```python
from build123d import *

# Parameters (mm, degrees)
BOSS_EXTRUDE1_DEPTH = 15
SKETCH5_R           = 10
CUT_EXTRUDE1_DEPTH  = 15


with BuildPart() as part:
    # Sketch3 → Boss-Extrude1 (new body)
    with BuildSketch(Plane(origin=(0, 0, 0), x_dir=(0, 0, -1), z_dir=(1, 0, 0))):
        Polygon((0, 0), (120, 0), (120, 80), (80, 80), (80, 40), (40, 40), (40, 80), (0, 80), align=None)
    extrude(amount=BOSS_EXTRUDE1_DEPTH)

    # Sketch5 → Cut-Extrude1 (cut)
    with BuildSketch(Plane.ZY):
        with Locations((-100, 20)):
            Circle(SKETCH5_R)
        with Locations((-20, 20)):
            Circle(SKETCH5_R)
    extrude(amount=-CUT_EXTRUDE1_DEPTH, mode=Mode.SUBTRACT)


solid = part.part
```
Read the model definition and answer for the solid it produces. Units are mm, in the model's axes. A direction names the side the tool comes from. Give positions to 0.01 mm unless a question says otherwise; leave off trailing zeros. Write each loop counter-clockwise with the first axis right and the second up, starting at its lowest first coordinate (ties: lowest second). Pieces come first, ordered by that corner, then holes. Notation, with made-up numbers: (49, 31.5) - (96, 31.5) arc R17 ccw to (96, 36.5) - close; hole circle Ø10 at (16, 66.5). An arc over 180 degrees is marked (long way). Write item = value, one per line. Start each with the question number.
Item 1: Find section B-B (y = 20). Give the vertices of the cut face in (x, z).
Item 2: Find the intervals of material crossed by probe 1 along Z at (x, y) = (12, 17); probe 2 along Y at (x, z) = (8.25, -20); probe 3 along Z at (x, y) = (10.25, 61), in increasing order. Write a range as [from, to].
Item 3: A tool of negligible diameter and unlimited length cuts with its end or side. For faces 4 (the flat face through (7, 60, -40)), 5 (the cylindrical face through (7.4, 26.76, -107.37)), from which of +Z, -Z, +X, -X, +Y, -Y can it reach the whole face along a straight path? Write none if from no direction.
Item 4: This flat-tipped pin is pushed along its axis until it touches: P1, Ø7.5, axis at x = 8, z = -58.5, coming from the +Y side. Where does it stop, or does it pass through?
Item 5: Find section A-A (y = 56.5). Give the vertices of the cut face in (x, z).
Item 6: Find section D-D (x = 2.75). Give the vertices of the cut face in (y, z), then the cut area to 3 significant figures.
Item 7: Find section C-C (z = -20). Give the vertices of the cut face in (x, y).
Item 8: The mould has two halves that part along Z. Classify faces 1 (the flat face through (7, 41, 0)), 2 (the flat face through (7, 40, -60)), 3 (the flat face through (15, 32, -59)): +Z half, -Z half, draft (parallel to the pull), parting line (faces both ways), or undercut.
Response:
q1.outline = (0, -120) - (15, -120) - (15, -110) - (0, -110) - close; (0, -90) - (15, -90) - (15, -30) - (0, -30) - close; (0, -10) - (15, -10) - (15, 0) - (0, 0) - close
q2.probe_1 = [-120, -109.54], [-90.46, -29.54], [-10.46, 0]
q2.probe_2 = [0, 10], [30, 80]
q2.probe_3 = [-120, -80], [-40, 0]
q3.face_4 = +X, -X, +Y
q3.face_5 = +X, -X
q4.P1 = 40
q5.outline = (0, -120) - (15, -120) - (15, -80) - (0, -80) - close; (0, -40) - (15, -40) - (15, 0) - (0, 0) - close
q6.outline = (0, -120) - (80, -120) - (80, -80) - (40, -80) - (40, -40) - (80, -40) - (80, 0) - (0, 0) - close; hole circle Ø20 at (20, -100); hole circle Ø20 at (20, -20)
q6.area = 7,370 mm²
q7.outline = (0, 0) - (15, 0) - (15, 10) - (0, 10) - close; (0, 30) - (15, 30) - (15, 80) - (0, 80) - close
q8.face_1 = +Z half
q8.face_2 = undercut
q8.face_3 = draft
